Part print with two shaded views. Sizes in mm from the minimum x, y, z corner. A direction names the side the tool comes from. Coordinates: 2 decimals unless noted, no trailing zeros. Write each loop counter-clockwise with the first axis right and the second up, starting at its lowest first coordinate (ties: lowest second). Pieces come first, ordered by that corner, then holes.
Q1. Band-saw the part on B-B, the plane y = 2.5. Write the cut outline in (x, z).
Q2. Band-saw the part on A-A, the plane z = 28.5. Write the cut outline in (x, y).
Q3. Pin check, flat tips, straight feed: P1, Ø1.5, axis at x = 11.5, y = 5, coming from the +Z side; P2, Ø11, axis at x = 12.5, z = 25.5, coming from the +Y side. Stop position of each tip, or through.
Q4. Pull direction X, two halves, no side cores. Call the marked faces 1, 2, 3 and 4: released by +X, released by -X, zero draft, split by the parting line, or undercut.
Q5. Which spindle directions (+Z, -Z, +X, -X, +Y, -Y) get a long thin tool onto all of the face, cutting with end or side? Do the marked faces 5 and 6. Say none if no direction does.
Q6. Band-saw the part on C-C, the plane x = 6.25. Write the cut outline in (y, z), plus the area to 3 significant figures.
Q7. Drill centre lines: probe 1 along X at (y, z) = (3.5, 26); probe 2 along Z at (x, y) = (12.5, 3.5). Where is each one in solid material? Low to high.
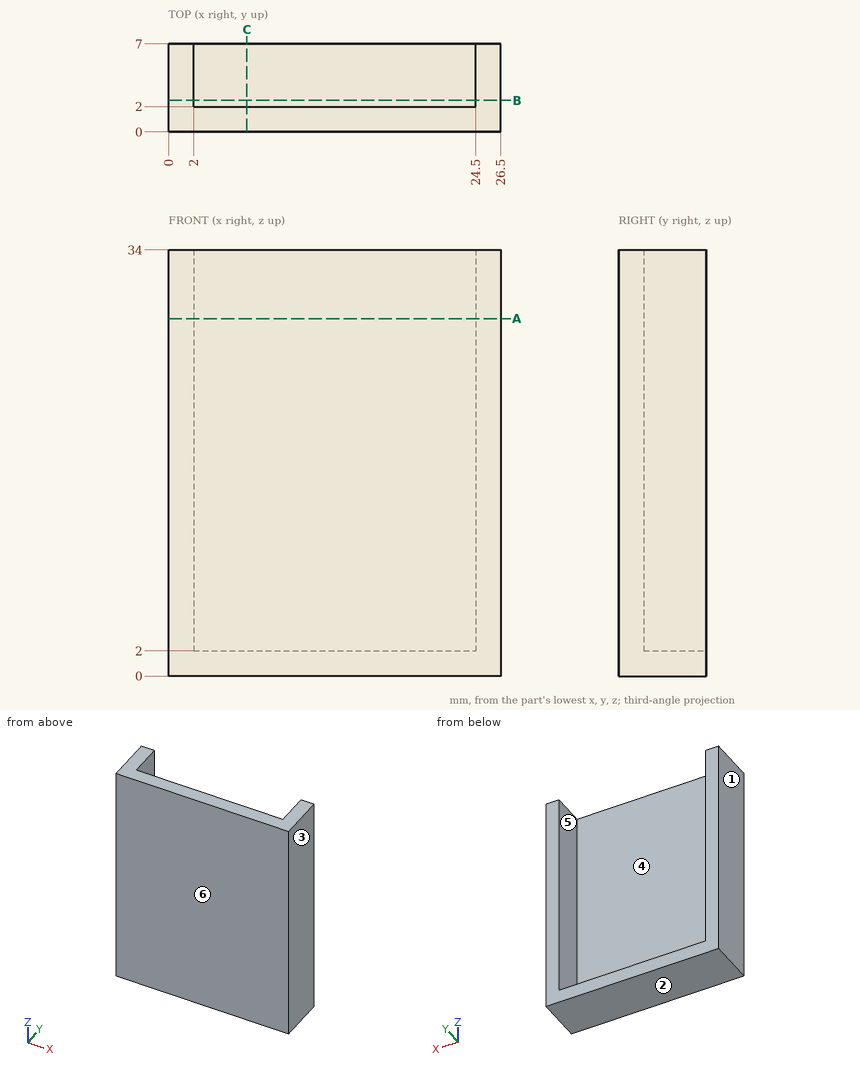
Answer sheet:
1. outline: (0, 0) - (26.5, 0) - (26.5, 34) - (24.5, 34) - (24.5, 2) - (2, 2) - (2, 34) - (0, 34) - close
2. outline: (0, 0) - (26.5, 0) - (26.5, 7) - (24.5, 7) - (24.5, 2) - (2, 2) - (2, 7) - (0, 7) - close
3. P1: stops at z = 2
3. P2: stops at y = 2
4. face 1: released by -X
4. face 2: zero draft
4. face 3: released by +X
4. face 4: undercut
5. face 5: +Z, +Y
5. face 6: +Z, -Z, +X, -X, -Y
6. outline: (0, 0) - (7, 0) - (7, 2) - (2, 2) - (2, 34) - (0, 34) - close
6. area: 78.0 mm2
7. probe 1: x = 0 to 2, 24.5 to 26.5
7. probe 2: z = 0 to 2
